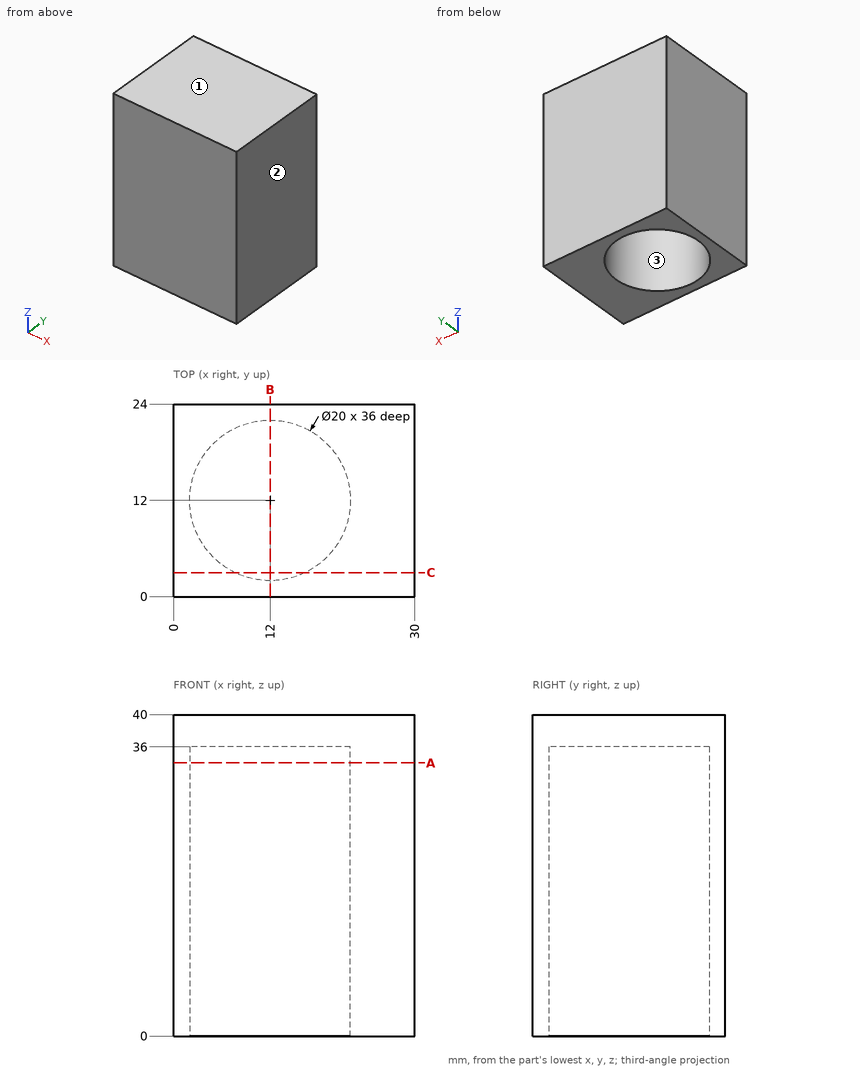
Here's the drawing with two shaded views (mm, measured from the low corner). I have some questions. Give positions to 0.01 mm unless a question says otherwise; leave off trailing zeros. Write each loop counter-clockwise with the first axis right and the second up, starting at its lowest first coordinate (ties: lowest second). Pieces come first, ordered by that corner, then holes. Notation, with made-up numbers: (-9, 64.25) -> (44, 64.25) arc R30 ccw to (44, 96.25) -> close; hole circle Ø9 at (16, -7.5). An arc over 180 degrees is marked (long way). Answer as a JSON object with one key per item and string values. Group by question number.
Item 1: Suppose I cut it at B-B (x = 12). Please give me the cut outline in (y, z).
Item 2: I'm going to push a flat-ended pin straight in: P1, Ø10, axis at x = 10, y = 12.5, coming from the -Z side. Where does the tip first touch, or does it pass through?
Item 3: Suppose I cut it at A-A (z = 34). Please give me the cut outline in (x, y), plus the area to 3 significant figures.
Item 4: Suppose I cut it at C-C (y = 3). Please give me the cut outline in (x, z), plus the area to 3 significant figures.
Item 5: Please list where these lines run through material, in increasing order: line 1 (Y direction, x = 12, z = 25.5); line 2 (X direction, y = 12, z = 13.5); line 3 (Z direction, x = 15.5, y = 8.5). Write a range as [from, to].
Item 6: We'd pull the mould along X, two halves only. Please class the marked faces 1, 2 and 3: +X half, -X half, draft (parallel to the pull), parting line (faces both ways), or undercut.
Findings:
{
 "1": {"outline": "(0, 0) -> (2, 0) -> (2, 36) -> (22, 36) -> (22, 0) -> (24, 0) -> (24, 40) -> (0, 40) -> close"},
 "2": {"P1": "stops at z = 36"},
 "3": {"outline": "(0, 0) -> (30, 0) -> (30, 24) -> (0, 24) -> close; hole circle Ø20 at (12, 12)", "area": "406 mm²"},
 "4": {"outline": "(0, 0) -> (7.64, 0) -> (7.64, 36) -> (16.36, 36) -> (16.36, 0) -> (30, 0) -> (30, 40) -> (0, 40) -> close", "area": "886 mm²"},
 "5": {"line 1": "y = [0, 2], [22, 24]", "line 2": "x = [0, 2], [22, 30]", "line 3": "z = [36, 40]"},
 "6": {"face 1": "draft", "face 2": "+X half", "face 3": "undercut"}
}
